Geometry: final body of the model. Coordinates: model frame, mm. A direction names the side the tool comes from. Give positions to 0.01 mm unless a question says otherwise; leave off trailing zeros. Order: outer loops, then holes, each group sorted by start corner. A loop starts at its lowest first (then second) coordinate and runs counter-clockwise, first axis right, second up. Notation, with made-up numbers: (-36.5, -12) - (0.5, -12) arc R25 cw to (0.5, 10) - close; hole circle Ø5 at (-22, 13.5). An arc over 180 degrees is marked (long way). Put each result on its own line as item: value. Start each with the question number.
1. Section C-C on z = 3.5. Count the separate pieces of the cut face and the enclosed holes in it, plus the area to 3 significant figures.
2. Section D-D on y = 18. Return the cut outline in (x, z).
3. First-contact query: P1, Ø10, axis at x = 47, y = 15.5, coming from the -Z side; P2, Ø1, axis at y = -28, z = 3, coming from the +X side; P3, Ø1.9, axis at x = 3, z = 3.5, coming from the -Y side (3 decimals); P4, Ø2.5, axis at y = -31.5, z = 3, coming from the +X side. Flat tips, straight axial feed; report the tip coordinate or a pass-through.
4. Ray query, line 1 along Y through (x, z) = (0, 5) (3 decimals); line 2 along Y through (x, z) = (-8, 2.5) (3 decimals); line 3 along Y through (x, z) = (-3.5, 2.25) (3 decimals). Return the intervals inside material, ascending. Write a range as from..to.
5. Mould query, pull axis X, two halves, no side actions, for faces 1 (the flat face through (-63.5, -44, 3)), 2 (the flat face through (35, 41.275, 3)), 3 (the cylindrical face through (-7.42, -34.59, 3.13)). Classes: pulls with the +X half, pulls with the -X half, needs draft (parallel to the pull), parting line crosses it, or undercut.
6. Set-up query: faces 4 (the flat face through (40.005, -31, 3)), 5 (the flat face through (67, -41.275, 3)), 6 (the flat face through (50.8, -44, 3)), 7 (the flat face through (2.121, 37, 3)). Return all of +Z, -Z, +X, -X, +Y, -Y with unobstructed straight access to the full face (end or side cutting, diameter ignored); none if empty.
7. Section B-B on x = -15.5. Return the cut outline in (y, z) (3 decimals), plus the area to 3 significant figures.
8. Section A-A on x = 7.75. Return the cut outline in (y, z) (3 decimals).
from build123d import *

# Parameters (mm, degrees)
SKETCH1_W           = 139.7
SKETCH1_H           = 82.55
BOSS_EXTRUDE1_DEPTH = 6.35
SKETCH2_W           = 12.7
SKETCH2_H           = 6.35
BOSS_EXTRUDE2_DEPTH = 6.35
CUT_EXTRUDE1_DEPTH  = 6.35
CUT_EXTRUDE8_DEPTH  = 6.35
CUT_EXTRUDE2_DEPTH  = 6.35
SKETCH5_R           = 6.254
SKETCH5_R_2         = 1.504
CUT_EXTRUDE9_DEPTH  = 6.35


with BuildPart() as part:
    # Sketch1 → Boss-Extrude1 (new body)
    with BuildSketch(Plane.XY):
        Rectangle(SKETCH1_W, SKETCH1_H)
    extrude(amount=BOSS_EXTRUDE1_DEPTH)

    # Sketch2 → Boss-Extrude2 (add)
    with BuildSketch(Plane(origin=(0, 0, 0), x_dir=(-1, 0, 0), z_dir=(0, 0, -1))):
        with Locations((-57.15, -44.45)):
            Rectangle(SKETCH2_W, SKETCH2_H)
        with Locations((-25.4, 44.45)):
            Rectangle(SKETCH2_W, SKETCH2_H)
    boss_extrude2 = extrude(amount=-BOSS_EXTRUDE2_DEPTH)

    # Sketch3 → Cut-Extrude1 (cut)
    with BuildSketch(Plane(origin=(0, 0, 0), x_dir=(-1, 0, 0), z_dir=(0, 0, -1))):
        Polygon((-46.5836, -41.275), (-46.5836, -32.512), (-48.895, -32.512), (-48.895, -29.337), (-46.5836, -29.337), (-46.5836, -26.035), (-42.3164, -26.035), (-42.3164, -29.337), (-40.005, -29.337), (-40.005, -32.512), (-42.3164, -32.512), (-42.3164, -41.275), align=None)
    cut_extrude1 = extrude(amount=-CUT_EXTRUDE1_DEPTH, mode=Mode.SUBTRACT)

    # Sketch7 → Cut-Extrude8 (cut)
    with BuildSketch(Plane(origin=(0, 0, 0), x_dir=(-1, 0, 0), z_dir=(0, 0, -1))):
        Polygon((-38.1, 41.275), (-69.85, -34.925), (-69.85, 41.275), align=None)
    cut_extrude8 = extrude(amount=-CUT_EXTRUDE8_DEPTH, mode=Mode.SUBTRACT)

    # Mirror2: Boss-Extrude2, Cut-Extrude8 across plane
    add(boss_extrude2.mirror(Plane(origin=(0, 0, 0), x_dir=(0, 0, 1), z_dir=(1, 0, 0))))
    add(cut_extrude8.mirror(Plane(origin=(0, 0, 0), x_dir=(0, 0, 1), z_dir=(1, 0, 0))), mode=Mode.SUBTRACT)

    # Mirror4: Cut-Extrude1 across plane
    add(cut_extrude1.mirror(Plane(origin=(0, 0, 0), x_dir=(0, 0, 1), z_dir=(1, 0, 0))), mode=Mode.SUBTRACT)

    # Sketch4 → Cut-Extrude2 (cut)
    with BuildSketch(Plane(origin=(0, 0, 0), x_dir=(-1, 0, 0), z_dir=(0, 0, -1))):
        Polygon((2.1209, 41.275), (-2.1209, 41.275), (-2.1209, 32.512), (-4.445, 32.512), (-4.445, 29.337), (-2.1209, 29.337), (-2.1209, 26.035), (2.1209, 26.035), (2.1209, 29.337), (4.445, 29.337), (4.445, 32.512), (2.1209, 32.512), align=None)
    extrude(amount=-CUT_EXTRUDE2_DEPTH, mode=Mode.SUBTRACT)

    # Sketch5 → Cut-Extrude9 (cut)
    with BuildSketch(Plane(origin=(0, 0, 0), x_dir=(-1, 0, 0), z_dir=(0, 0, -1))):
        with Locations((0, -26.7)):
            Circle(SKETCH5_R)
        with Locations((-15.5, -19.7)):
            Circle(SKETCH5_R_2)
        with Locations((-7.75, -6.276606241)):
            Circle(SKETCH5_R_2)
        with Locations((7.75, -6.276606241)):
            Circle(SKETCH5_R_2)
        with Locations((15.5, -19.7)):
            Circle(SKETCH5_R_2)
        with Locations((7.75, -33.123393759)):
            Circle(SKETCH5_R_2)
        with Locations((-7.75, -33.123393759)):
            Circle(SKETCH5_R_2)
    extrude(amount=-CUT_EXTRUDE9_DEPTH, mode=Mode.SUBTRACT)


solid = part.part
Resolved:
1. separate pieces: 1
1. enclosed holes: 7
1. area: 9,030 mm^2
2. outline: (-47.8, 0) - (47.8, 0) - (47.8, 6.35) - (-47.8, 6.35) - close
3. P1: z = 0
3. P2: x = 67.17
3. P3: y = -41.275
3. P4: x = 68.94
4. line 1: -41.275..-32.954, -20.446..26.035
4. line 2: -41.275..-34.606, -31.64..-7.76, -4.794..41.275
4. line 3: -41.275..-31.883, -21.517..29.337, 32.512..41.275
5. face 1: pulls with the -X half
5. face 2: needs draft
5. face 3: undercut
6. face 4: +Z, -Z
6. face 5: +Z, -Z, +X, -Y
6. face 6: +Z, -Z, -Y
6. face 7: +Z, -Z, +Y
7. outline: (-41.275, 0) - (-21.204, 0) - (-21.204, 6.35) - (-41.275, 6.35) - close; (-18.196, 0) - (41.275, 0) - (41.275, 6.35) - (-18.196, 6.35) - close
7. area: 505 mm^2
8. outline: (-41.275, 0) - (-34.627, 0) - (-34.627, 6.35) - (-41.275, 6.35) - close; (-31.619, 0) - (-7.781, 0) - (-7.781, 6.35) - (-31.619, 6.35) - close; (-4.773, 0) - (41.275, 0) - (41.275, 6.35) - (-4.773, 6.35) - close
